```python
from build123d import *

# Parameters (mm, degrees)
F0_W         = 60.96
F0_H         = 104.14
F1_DEPTH     = 10.414
F3_R         = 17.78
F3_R_2       = 7.62
F4_DEPTH     = 0.254
F2_W         = 55.1793798804
F2_H         = 38.1
F5_DEPTH     = 0.254
F6_R         = 2.3165887379
F7_DEPTH     = 25.4
F8_W         = 14.3902888522
F8_H         = 3.1658638036
F9_DEPTH     = 0.254
F10_W        = 20.8778993692
F10_H        = 2.1391292103
F11_DEPTH    = 25.4
F12_R        = 5.08
F13_T1_DEPTH = 35.814
F14_R        = 5.08
F15_R        = 5.08


# Not quite as in the source:
# - a fillet or chamfer that OpenCascade refuses, or shapes differently, is made with other operations: its cross-section is extruded or revolved along the edge and cut away or added


with BuildPart() as f1:
    # F0 (on Front) → F1 (new body)
    with BuildSketch(Plane.XZ):
        with Locations((-7.5916079104, 5.2405595779)):
            Rectangle(F0_W, F0_H)
    extrude(amount=F1_DEPTH)

    # F3 (on face) → F4 (join)
    with BuildSketch(Plane.XZ.offset(10.414)):
        with Locations((-6.9598197006, -16.3494404221)):
            Circle(F3_R)
        with Locations((-6.9598197006, -16.3494404221)):
            Circle(F3_R_2, mode=Mode.SUBTRACT)
    extrude(amount=F4_DEPTH)

    # F2 (on face) → F5 (join)
    with BuildSketch(Plane.XZ.offset(10.414)):
        with Locations((-7.2018355131, 31.9105595779)):
            Rectangle(F2_W, F2_H)
    extrude(amount=F5_DEPTH)

    # F6 (on face) → F7 (cut)
    with BuildSketch(Plane.XY.offset(57.3105595779)):
        with Locations((-31.0040302575, -2.9813330621)):
            Circle(F6_R)
    extrude(amount=-F7_DEPTH, mode=Mode.SUBTRACT)

    # F8 (on face) → F9 (join)
    with BuildSketch(Plane.XY.offset(57.3105595779)):
        with Locations((9.3301092274, -3.0921686557)):
            Rectangle(F8_W, F8_H)
    extrude(amount=F9_DEPTH)

    # F10 (on face) → F11 (cut)
    with BuildSketch(Plane(origin=(0, 0, -46.8294404221), x_dir=(1, 0, 0), z_dir=(0, 0, -1))):
        with Locations((-6.7444174783, 3.3060612623)):
            Rectangle(F10_W, F10_H)
    extrude(amount=-F11_DEPTH, mode=Mode.SUBTRACT)

    # F12
    f12_edges = [f1.edges().sort_by_distance(p)[0] for p in [
        (-38.071608, -5.207, -46.82944),
    ]]
    fillet(f12_edges, radius=F12_R)

    # F13: fillet of radius 5.08 on 1 edges, made by hand

    # F13_s2 → F13_t1 (cut)
    with BuildSketch(Plane.XZ.offset(-12.7)):
        with BuildLine():
            ThreePointArc((-38.0716079104, 52.2305595779), (-36.5837103588, 55.8226620264), (-32.9916079104, 57.3105595779))
            Line((-32.9916079104, 57.3105595779), (-38.0716079104, 57.3105595779))
            Line((-38.0716079104, 57.3105595779), (-38.0716079104, 52.2305595779))
        make_face()
    extrude(amount=F13_T1_DEPTH, mode=Mode.SUBTRACT)

    # F14
    f14_edges = [f1.edges().sort_by_distance(p)[0] for p in [
        (22.888392, -5.207, -46.82944),
    ]]
    fillet(f14_edges, radius=F14_R)

    # F15
    f15_edges = [f1.edges().sort_by_distance(p)[0] for p in [
        (22.888392, -5.207, 57.31056),
    ]]
    fillet(f15_edges, radius=F15_R)


solid = f1.part
```
Check sheet for the modelled part. Datum: model origin and axes. Units: mm. A direction names the side the tool comes from. Coordinates: 2 decimals unless noted, no trailing zeros. Loops run counter-clockwise (first coordinate to the right, second up) from the corner with the lowest first, then second, coordinate; pieces in that order, holes last.
1) Gauge pin test, flat ends, axial feed: pin 1 (5 mm diameter, centred on x = -30.5, y = -2, fed in from +Z); pin 2 (4.5 mm diameter, centred on x = -8.5, z = -15, fed in from -Y). Record the tip position at first contact, or that the pin passes through.
2) Access from +Z, -Z, +X, -X, +Y, -Y to the whole of each face (thin tool, end or side, straight path). Record for faces 5 (the face through (-31, -3, 31.911)), 6 (the face through (-7, -4.376, -34)), 7 (the face through (-38.072, -5, 5)), 8 (the face through (-7, -10.414, -16)).
3) Release check for a two-part mould opening along Y. For faces 1 (the face through (3.695, -3, -34)), 2 (the face through (-8, -10.668, 32)), 3 (the face through (-8, 0, 6)), 4 (the face through (9, -3, 57.565)) record: released by +Y, released by -Y, zero draft, split by the parting line, or undercut.
4) Sectioned sample at A-A (x = -8). Record the boundary of the cut face in (y, z).
5) Material ranges on probe 1 along Y at (x, z) = (-19.5, -3); probe 2 along X at (y, z) = (-3.25, -25); probe 3 along Y at (x, z) = (-10, -21.5), recorded low to high.
6) Sectioned sample at C-C (z = 2.5). Record the boundary of the cut face in (x, y).
7) Sectioned sample at D-D (x = -16). Record the boundary of the cut face in (y, z), and give its area (3 significant figures).
8) Sectioned sample at B-B (z = 33). Record the boundary of the cut face in (x, y), and give its area (3 significant figures).
Check sheet entries:
1. pin 1: stops at z = 57.31
1. pin 2: stops at y = -10.41
2. face 5: +Z
2. face 6: -Z
2. face 7: +Z, -Z, -X, +Y, -Y
2. face 8: -Y
3. face 1: undercut
3. face 2: released by -Y
3. face 3: released by +Y
3. face 4: zero draft
4. outline: (-10.67, -34.1) - (-10.41, -34.1) - (-10.41, -46.83) - (-4.38, -46.83) - (-4.38, -21.43) - (-2.24, -21.43) - (-2.24, -46.83) - (0, -46.83) - (0, 57.31) - (-10.41, 57.31) - (-10.41, 50.96) - (-10.67, 50.96) - (-10.67, 12.86) - (-10.41, 12.86) - (-10.41, 1.4) - (-10.67, 1.4) - (-10.67, -8.8) - (-10.41, -8.8) - (-10.41, -23.9) - (-10.67, -23.9) - close
5. probe 1: y = -10.41 to 0
5. probe 2: x = -38.07 to -17.18, 3.69 to 22.89
5. probe 3: y = -10.41 to -4.38, -2.24 to 0
6. outline: (-38.07, -10.41) - (22.89, -10.41) - (22.89, 0) - (-38.07, 0) - close
7. outline: (-10.67, -31.66) - (-10.41, -31.66) - (-10.41, -46.83) - (-4.38, -46.83) - (-4.38, -21.43) - (-2.24, -21.43) - (-2.24, -46.83) - (0, -46.83) - (0, 57.31) - (-10.41, 57.31) - (-10.41, 50.96) - (-10.67, 50.96) - (-10.67, 12.86) - (-10.41, 12.86) - (-10.41, -1.04) - (-10.67, -1.04) - close
7. area: 1,050 mm2
8. outline: (-38.07, -10.41) - (-34.79, -10.41) - (-34.79, -10.67) - (20.39, -10.67) - (20.39, -10.41) - (22.89, -10.41) - (22.89, 0) - (-38.07, 0) - close; hole circle Ø4.63 at (-31, -2.98)
8. area: 632 mm2
